CAD build for the part. Positions are in the model's coordinates, mm. Face numbers are marked on the shaded views. A direction names the side the tool comes from. Coordinates: 2 decimals unless noted, no trailing zeros. Order: outer loops, then holes, each group sorted by start corner. A loop starts at its lowest first (then second) coordinate and runs counter-clockwise, first axis right, second up. Notation, with made-up numbers: (60, 5) - (97, 5) arc R17 ccw to (97, 33) - close; hole circle Ø1 at (51.25, 60). An arc over 180 degrees is marked (long way). Write each question's results on one line, items separated by ' | '. Start each with the question number.
Q1. Pull direction X, two halves, no side cores. Call the marked faces 3, 4, 5 and 6: released by +X, released by -X, zero draft, split by the parting line, or undercut.
Q2. Which spindle directions (+Z, -Z, +X, -X, +Y, -Y) get a long thin tool onto all of the face, cutting with end or side? Do the marked faces 1 and 2. Say none if no direction does.
Q3. Wall check: probe 1 along Y at (x, z) = (-15, 1.45); probe 2 along X at (y, z) = (15, 2.9); probe 3 along X at (y, z) = (-33.3, 12.5). Give the ranges that are in metal, low to high.
Q4. Band-saw the part on D-D, the plane x = 8. Write the cut outline in (y, z), then the cut area to 3 significant figures.
Q5. Band-saw the part on B-B, the plane z = 12.5. Write the cut outline in (x, y), then the cut area to 3 significant figures.
Q6. Band-saw the part on A-A, the plane y = 0. Write the cut outline in (x, z), then the cut area to 3 significant figures.
Q7. Pin check, flat tips, straight feed: P1, Ø5, axis at x = 11.5, z = 10, coming from the +Y side; P2, Ø8.5, axis at x = -11.5, z = 14, coming from the +Y side; P3, Ø4.5, axis at x = 15, y = -15, coming from the +Z side; P4, Ø6, axis at y = 9.5, z = 6.5, coming from the -X side. Stop position of each tip, or through.
Q8. Band-saw the part on C-C, the plane y = 15. Write the cut outline in (x, z).
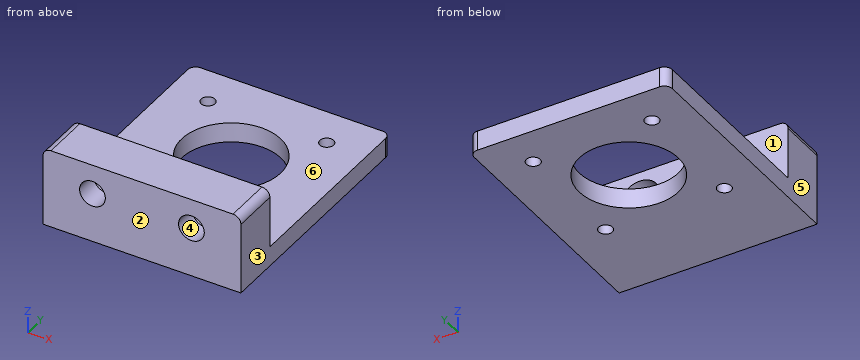
Autodesk Inventor part; units mm, degrees
ref_plane "Work Plane1" through (0, -37, 0) normal (0, 1, 0) x (-1, 0, 0)
ref_plane "YZ Plane" through (0, 0, 0) normal (1, 0, 0) x (0, 1, 0)
ref_plane "XY Plane" through (0, 0, 0) normal (0, 0, 1) x (1, 0, 0)
sketch "Sketch1" plane through (0, 0, 0) normal (0, 0, 1) x (1, 0, 0)
  circle A0 centre (0, 0) radius 12.5
  line L0 (25, -25) -> (-25, -25)
  line L1 (-25, -25) -> (-25, 25)
  line L2 (-25, 25) -> (25, 25)
  line L3 (25, 25) -> (25, -25)
  line L4 (25, -25) -> (-25, 25) construction
  line L5 (-25, -25) -> (25, 25) construction
  point P0 (-15, 15)
  point P1 (15, 15)
  point P2 (-15, -15)
  point P3 (15, -15)
  dimension "d0" = 25
  dimension "d1" = 50
  dimension "d2" = 50
  dimension "d5" = 30
  dimension "d8" = 30
extrude "Extrusion1" add sketch "Sketch1" along normal blind 5
hole "Hole1" at (-15, 15, 0) at (15, 15, 0) at (-15, -15, 0) at (15, -15, 0) direction (0, 0, 1) diameter 3.5 end through all
ref_plane "Work Plane1" through (0, -37, 0) normal (0, 1, 0) x (-1, 0, 0)
sketch "Sketch2" plane through (0, -37, 0) normal (0, 1, 0) x (-1, 0, 0)
  line L0 (-25, 0) -> (25, 0)
  line L1 (-25, 0) -> (-25, 5)
  line L2 (25, 0) -> (-25, 0)
  line L3 (-25, 0) -> (-25, 20)
  line L4 (-25, 20) -> (25, 20)
  line L5 (25, 20) -> (25, 0)
  point P0 (0, 0)
  point P1 (12.5, 12.5)
  point P2 (-12.5, 12.5)
  dimension "d21" = 20
  dimension "d24" = 25
  dimension "d46" = 12.5
extrude "Extrusion2" add sketch "Sketch2" along normal up to surface (12 mm away)
hole "Hole2" at (12.5, -37, 12.5) at (-12.5, -37, 12.5) direction (0, 1, 0) diameter 6.5 end through all
fillet "Fillet1" radius 2 4 edges at (25, 25, 2.5) (-25, 25, 2.5) (25, -31, 20) (-25, -31, 20)
sketch "Sketch5" plane through (-25, -25, 5) normal (0, 1, 0) x (1, 0, 0)
  point P0 (25, 5)
  point P1 (12.5, -7.5)
  point P2 (37.5, -7.5)
hole "Hole4" at (-12.5, -25, 12.5) at (12.5, -25, 12.5) direction (0, -1, 0) diameter 10.5 depth 6.2
properties part number "mirror-bracket"
Results below:
1) face 3: released by +X | face 4: undercut | face 5: released by -X | face 6: zero draft
2) face 1: +Z, +X, -X, +Y | face 2: +Z, -Z, +X, -X, -Y
3) probe 1: y = -37 to -16.75, -13.25 to 13.25, 16.75 to 25 | probe 2: x = -25 to -16.75, -13.25 to 13.25, 16.75 to 25 | probe 3: x = -25 to -15.75, -9.25 to 9.25, 15.75 to 25
4) outline: (-37, 0) - (-9.6, 0) - (-9.6, 5) - (-25, 5) - (-25, 9.8) - (-31.2, 9.8) - (-31.2, 15.2) - (-25, 15.2) - (-25, 20) - (-37, 20) - close; (9.6, 0) - (25, 0) - (25, 5) - (9.6, 5) - close | area: 360 mm²
5) outline: (-25, -37) - (-15.75, -37) - (-15.75, -31.2) - (-17.75, -31.2) - (-17.75, -25) - (-25, -25) - close; (-9.25, -37) - (9.25, -37) - (9.25, -31.2) - (7.25, -31.2) - (7.25, -25) - (-7.25, -25) - (-7.25, -31.2) - (-9.25, -31.2) - close; (15.75, -37) - (25, -37) - (25, -25) - (17.75, -25) - (17.75, -31.2) - (15.75, -31.2) - close | area: 394 mm²
6) outline: (-25, 0) - (-12.5, 0) - (-12.5, 5) - (-25, 5) - close; (12.5, 0) - (25, 0) - (25, 5) - (12.5, 5) - close | area: 125 mm²
7) P1: stops at y = -31.2 | P2: stops at y = -25 | P3: stops at z = 5 | P4: stops at x = -25
8) outline: (-25, 0) - (-16.75, 0) - (-16.75, 5) - (-25, 5) - close; (-13.25, 0) - (13.25, 0) - (13.25, 5) - (-13.25, 5) - close; (16.75, 0) - (25, 0) - (25, 5) - (16.75, 5) - close
